Job drawing, mm, ordinate dimensions from the low corner. One solid piece. A direction names the side the tool comes from. Coordinates: 2 decimals unless noted, no trailing zeros. Order: outer loops, then holes, each group sorted by start corner. A loop starts at its lowest first (then second) coordinate and runs counter-clockwise, first axis right, second up. Notation, with made-up numbers: M -12,41 L 6,41 A23 ccw 6,67 Z; hole C 5.5,7 d9. An arc over 180 degrees is marked long. Write item = value, one per line.
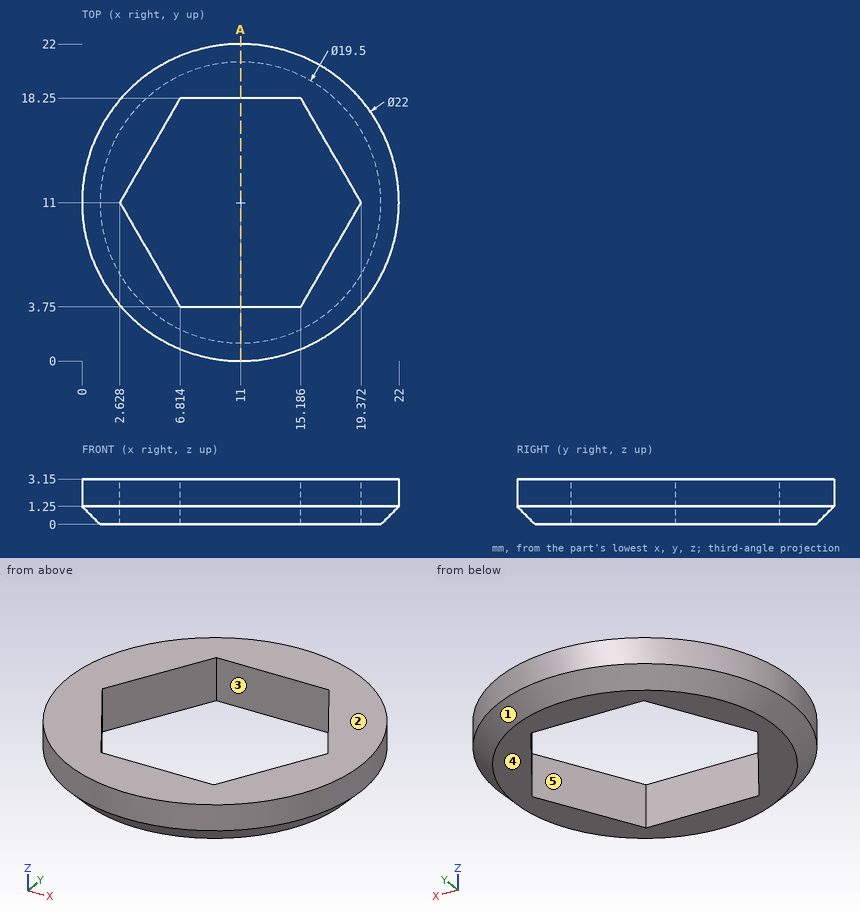
(1) Wall check: line 1 (X direction, y = 9.5, z = 1.05) (1 decimal); line 2 (Y direction, x = 18.75, z = 0.5) (1 decimal); line 3 (Y direction, x = 3.25, z = 1.05) (1 decimal). Give the ranges that are in metal, low to high. Write a range as from..to.
Evaluation:
line_1 = 0.3..3.5, 18.5..21.7
line_2 = 4.3..9.9, 12.1..17.7
line_3 = 3.5..9.9, 12.1..18.5
(2) Slice it at A-A, the plane x = 11. Write the cut outline in (y, z).
Evaluation:
outline = M 0,1.25 L 1.25,0 L 3.75,0 L 3.75,3.15 L 0,3.15 Z; M 18.25,0 L 20.75,0 L 22,1.25 L 22,3.15 L 18.25,3.15 Z
(3) Tool access for the marked faces 4 and 5: list every direction of +Z, -Z, +X, -X, +Y, -Y with a clear straight run to the whole face (end or side of a thin tool).
Evaluation:
face_4 = -Z, +X, -X, +Y, -Y
face_5 = +Z, -Z
(4) Pull direction X, two halves, no side cores. Call the marked faces 1, 2 and 3: +X half, -X half, draft (parallel to the pull), parting line (faces both ways), or undercut.
Evaluation:
face_1 = parting line
face_2 = draft
face_3 = undercut
(5) Pin check, flat tips, straight feed: pin 1 Ø3 at (x, y) = (7.5, 12.5) entering from -Z; pin 2 Ø1.5 at (x, z) = (16.5, 1.5) entering from -Y; pin 3 Ø1.6 at (x, z) = (9, 1.5) entering from +Y; pin 4 Ø1.6 at (x, z) = (9, 1.5) entering from -Y. Stop position of each tip, or through.
Evaluation:
pin_1 = through
pin_2 = 1.08
pin_3 = 21.93
pin_4 = 0.07
